Can you work these out from the model? Positions are in its coordinate system, mm. A direction names the side the tool comes from. Coordinates: 2 decimals unless noted, no trailing zeros. Order: outer loops, then holes, each group sorted by start corner. A loop starts at its lowest first (then second) coordinate and runs counter-clockwise, first axis right, second up. Notation, with made-up numbers: (37, 62) - (69, 62) arc R27 ccw to (69, 88) - close; hole circle Ø11 at (25.25, 65). An arc over 180 degrees is marked (long way). Return JSON: item names as keys, results as strings. Group by question number.
1) Imagine slicing it at C-C (z = -2.5). Write out the boundary of the cut face in (x, y), and give its area (3 significant figures).
2) If I drill on line 1 along Y through (x, z) = (0, -2.5); line 2 along Y through (x, z) = (0, 3.5); line 3 along X through (y, z) = (-6.25, 5.25), over which ranges is the centre line in solid material (lowest first)?
3) If we mould it in two halves opening along Y, with no side actions, what happens to faces 1 (the face through (5, 9, 4.5)), 2 (the face through (2.195, -9.884, 6.094)), 3 (the face through (-4.57, 7.167, 0.775))? For each: pulls with the +Y half, pulls with the -Y half, needs draft (parallel to the pull), parting line crosses it, or undercut.
4) Which directions (+Z, -Z, +X, -X, +Y, -Y) give clear straight access to the entire face, cutting with the end or side of a thin tool? Please do faces 4 (the face through (2.17, -9.76, 4.05)), 5 (the face through (2.17, -9.76, -3.18)), 6 (the face through (-4.5, -7.4, 6.2)).
5) For pin 1 Ø6 at (x, z) = (-3.5, -3) entering from -Y; pin 2 Ø6 at (x, z) = (4, 0.5) entering from -Y; pin 3 Ø1 at (y, z) = (-6, 0.5) entering from +X, each with a flat end and sliding along its axis, tell me the tip position at first contact or that it passes through.
6) Imagine slicing it at D-D (z = -0.75). Write out the boundary of the cut face in (x, y), and give its area (3 significant figures).
```python
from build123d import *

# Parameters (mm, degrees)
F3_D = 17


with BuildPart() as f1:
    # F0 (on Front) → F1 (revolve)
    with BuildSketch(Plane.XZ):
        Polygon((-10, -1.820884), (-10, -4.5), (0, -4.5), (0, 6.2), (-10, 6.2), (-12, 4.5), (-10, 4.5), (-10, 3.607264), (-10.25, 3.607264), (-10, 2.250227), (-10.25, 2.250227), (-10, 0.89319), (-10.25, 0.89319), (-10, -0.463847), (-10.25, -0.463847), align=None)
    revolve(axis=Axis((0, 0, 0.85), (0, 0, -1)))

    # F3 (through all)
    with Locations(Plane.XY.offset(6.2)):
        with Locations((0, 0)):
            Hole(F3_D / 2)


solid = f1.part
```
Calculated:
{
 "1": {"outline": "circle Ø20 at (0, 0); hole circle Ø17 at (0, 0)", "area": "87.2 mm2"},
 "2": {"line 1": "-10 to -8.5, 8.5 to 10", "line 2": "-10.23 to -8.5, 8.5 to 10.23", "line 3": "-9.19 to -5.76, 5.76 to 9.19"},
 "3": {"face 1": "needs draft", "face 2": "parting line crosses it", "face 3": "undercut"},
 "4": {"face 4": "none", "face 5": "-Z", "face 6": "+Z, +X, -X, +Y, -Y"},
 "5": {"pin 1": "y = -10.08", "pin 2": "y = -10.2", "pin 3": "x = 8.58"},
 "6": {"outline": "circle Ø20.39 at (0, 0); hole circle Ø17 at (0, 0)", "area": "99.7 mm2"}
}
